```python
from build123d import *

# Parameters (mm, degrees)
SKETCH1_W           = 50.8
SKETCH1_H           = 25.4
SKETCH1_W_2         = 47.498
SKETCH1_H_2         = 22.098
BOSS_EXTRUDE1_DEPTH = 330
SKETCH2_R           = 3.300000004
CUT_EXTRUDE2_DEPTH  = 26.4
CUT_EXTRUDE3_DEPTH  = 8.89


with BuildPart() as part:
    # Sketch1 → Boss-Extrude1 (new body)
    with BuildSketch(Plane.XY):
        with Locations((11.394392523, 4.86635514)):
            Rectangle(SKETCH1_W, SKETCH1_H)
        with Locations((11.394392523, 4.86635514)):
            Rectangle(SKETCH1_W_2, SKETCH1_H_2, mode=Mode.SUBTRACT)
    extrude(amount=BOSS_EXTRUDE1_DEPTH)

    # Sketch2 → Cut-Extrude2 (cut, through all)
    with BuildSketch(Plane(origin=(0, 17.56635514, 0), x_dir=(1, 0, 0), z_dir=(0, 1, 0))):
        with Locations((-2.423312001, -292.04835777)):
            Circle(SKETCH2_R)
        with Locations((22.930034754, -289.766295475)):
            Circle(SKETCH2_R)
        with Locations((25.212097048, -315.11964223)):
            Circle(SKETCH2_R)
        with Locations((-0.141249707, -317.401704525)):
            Circle(SKETCH2_R)
    extrude(amount=-CUT_EXTRUDE2_DEPTH, mode=Mode.SUBTRACT)

    # Sketch4 → Cut-Extrude3 (cut)
    with BuildSketch(Plane(origin=(0, 17.56635514, 0), x_dir=(1, 0, 0), z_dir=(0, 1, 0))):
        with BuildLine():
            ThreePointArc((14.950392523, -303.584), (11.394392523, -300.028), (7.838392523, -303.584))
            Line((7.838392523, -303.584), (7.838392523, -330))
            Line((7.838392523, -330), (14.950392523, -330))
            Line((14.950392523, -330), (14.950392523, -303.584))
        make_face()
    extrude(amount=-CUT_EXTRUDE3_DEPTH, mode=Mode.SUBTRACT)


solid = part.part
```
CAD build for the part. Positions are in the model's coordinates, mm. A direction names the side the tool comes from. Coordinates: 2 decimals unless noted, no trailing zeros. Write each loop counter-clockwise with the first axis right and the second up, starting at its lowest first coordinate (ties: lowest second). Pieces come first, ordered by that corner, then holes. Notation, with made-up numbers: (42.25, 82) -> (62.25, 82) arc R32 ccw to (62.25, 109) -> close; hole circle Ø4 at (-7, -2.5). An arc over 180 degrees is marked (long way). Return JSON: item names as keys, results as strings. Group by question number.
Q1. Cut at B-B, the plane z = 112. Give the cut face in (x, y).
Q2. Cut at A-A, the plane x = 32. Give the cut face in (y, z).
Q3. Flat gauge pins, fed straight in: pin 1 (4 mm diameter, centred on x = -0.14, z = 317.4, fed in from -Y); pin 2 (7.5 mm diameter, centred on x = 25.21, z = 315.12, fed in from -Y). Where does each tip first touch, or does it go through?
Q4. Drill centre lines: line 1 (X direction, y = 15.75, z = 295); line 2 (Y direction, x = 13, z = 15); line 3 (Y direction, x = 13, z = 306.5). Where is each one in solid material? Low to high.
Q5. Which spindle directions (+Z, -Z, +X, -X, +Y, -Y) get a long thin tool onto all of the face, cutting with end or side? Do faces 1 (the face through (-0.857, -6.997, 320.623)), 2 (the face through (35.143, 5, 163)). Say none if no direction does.
Q6. Cut at C-C, the plane y = 5. Give the cut face in (x, z), then the cut area to 3 significant figures.
Q7. Pull direction Y, two halves, no side cores. Call faces 3 (the face through (11, 17.566, 163)), 4 (the face through (11, -7.834, 163)), 5 (the face through (9.4, -6.4, 0)), 6 (the face through (11, 15.915, 163)): released by +Y, released by -Y, zero draft, split by the parting line, or undercut.
Returned:
{
 "1": {"outline": "(-14.01, -7.83) -> (36.79, -7.83) -> (36.79, 17.57) -> (-14.01, 17.57) -> close; hole (-12.35, -6.18) -> (35.14, -6.18) -> (35.14, 15.92) -> (-12.35, 15.92) -> close"},
 "2": {"outline": "(-7.83, 0) -> (-6.18, 0) -> (-6.18, 330) -> (-7.83, 330) -> close; (15.92, 0) -> (17.57, 0) -> (17.57, 330) -> (15.92, 330) -> close"},
 "3": {"pin 1": "passes through", "pin 2": "stops at y = -7.83"},
 "4": {"line 1": "x = -14.01 to -12.35, 35.14 to 36.79", "line 2": "y = -7.83 to -6.18, 15.92 to 17.57", "line 3": "y = -7.83 to -6.18"},
 "5": {"face 1": "+Y, -Y", "face 2": "+Z, -Z"},
 "6": {"outline": "(-14.01, 0) -> (-12.35, 0) -> (-12.35, 330) -> (-14.01, 330) -> close; (35.14, 0) -> (36.79, 0) -> (36.79, 330) -> (35.14, 330) -> close", "area": "1,090 mm2"},
 "7": {"face 3": "released by +Y", "face 4": "released by -Y", "face 5": "zero draft", "face 6": "undercut"}
}
